Build history of the part. All positions in model axes, mm. A direction names the side the tool comes from. Round coordinates to 2 decimals unless told otherwise and drop trailing zeros. Loops run counter-clockwise (first coordinate to the right, second up) from the corner with the lowest first, then second, coordinate; pieces in that order, holes last.
from build123d import *

# Parameters (mm, degrees)
SKETCH1_W               = 150
SKETCH1_H               = 150
BOSS_EXTRUDE1_DEPTH     = 10
CUT_EXTRUDE1_DEPTH      = 3.1
CUT_EXTRUDE1_DEPTH_BACK = 3.1
CUT_EXTRUDE2_DEPTH      = 8.2
CUT_EXTRUDE2_DEPTH_BACK = 2
SKETCH4_W               = 24.2
SKETCH4_H               = 2


with BuildPart() as part:
    # Sketch1 → Boss-Extrude1 (new body)
    with BuildSketch(Plane(origin=(0, 0, 0), x_dir=(1, 0, 0), z_dir=(0, 1, 0))):
        Rectangle(SKETCH1_W, SKETCH1_H)
    extrude(amount=BOSS_EXTRUDE1_DEPTH)

    # Sketch3 → Cut-Extrude1 (cut, two sides: drawn at the far end of the back side and taken through both)
    with BuildSketch(Plane(origin=(0, 0, 0), x_dir=(0, -1, 0), z_dir=(0.7071067811865488, 0, 0.7071067811865464)).offset(-CUT_EXTRUDE1_DEPTH_BACK)):
        with BuildLine():
            Line((-4, -68.177876041), (-6, -68.177876041))
            ThreePointArc((-6, -68.177876041), (-6.294051831, -69.777876041), (-6, -71.377876041))
            Line((-6, -71.377876041), (-6, -75.277876041))
            Line((-6, -75.277876041), (-8, -75.277876041))
            Line((-8, -75.277876041), (-8, -65.077876041))
            Line((-8, -65.077876041), (-10, -65.077876041))
            Line((-10, -65.077876041), (-10, -89.277876041))
            Line((-10, -89.277876041), (-8, -89.277876041))
            Line((-8, -89.277876041), (-8, -83.277876041))
            Line((-8, -83.277876041), (-4, -83.277876041))
            Line((-4, -83.277876041), (-4, -71.377876041))
            ThreePointArc((-4, -71.377876041), (-3.705948169, -69.777876041), (-4, -68.177876041))
        make_face()
    extrude(amount=CUT_EXTRUDE1_DEPTH + CUT_EXTRUDE1_DEPTH_BACK, mode=Mode.SUBTRACT)

    # Sketch4 → Cut-Extrude2 (cut, two sides: drawn at the far end of the back side and taken through both)
    with BuildSketch(Plane(origin=(-2.192031022, 0, -2.192031022), x_dir=(0.7071067811865465, 0, -0.7071067811865487), z_dir=(0.7071067811865487, 0, 0.7071067811865465)).offset(-CUT_EXTRUDE2_DEPTH_BACK)):
        with Locations((-77.177876041, 9)):
            Rectangle(SKETCH4_W, SKETCH4_H)
    extrude(amount=CUT_EXTRUDE2_DEPTH + CUT_EXTRUDE2_DEPTH_BACK, mode=Mode.SUBTRACT)

    # Sketch5 → Revolve1 (revolve)
    with BuildSketch(Plane(origin=(0, 0, 0), x_dir=(0, -1, 0), z_dir=(0.7071067811865488, 0, 0.7071067811865464)), mode=Mode.PRIVATE) as revolve1_sk:
        with BuildLine():
            Line((-10, 46.066017178), (-35, 46.066017178))
            ThreePointArc((-35, 46.066017178), (-29.607626316, 53.030055538), (-21.31365255, 50.066017178))
            Line((-21.31365255, 50.066017178), (-10, 50.066017178))
            Line((-10, 50.066017178), (-10, 46.066017178))
        make_face()
    revolve(revolve1_sk.sketch.rotate(Axis((32.573593129, 36.96807126, -32.573593129), (0, -1, 0)), 135), axis=Axis((32.573593129, 36.96807126, -32.573593129), (0, -1, 0)))


solid = part.part
(1) Slice it at B-B on z = -6. List the corners of the cut face in (x, y), plus the area to 3 significant figures.
Responses:
outline: (-75, 0) - (75, 0) - (75, 10) - (-75, 10) - close
area: 1,500 mm2
(2) Pull direction X, two halves, no side cores. Call faces 4 (the face through (-75, 5, 1)), 5 (the face through (-49.355, 6.294, 49.294)), 6 (the face through (75, 5, 1)): +X half, -X half, draft (parallel to the pull), parting line (faces both ways), or undercut.
Responses:
face 4: -X half
face 5: undercut
face 6: +X half
(3) Slice it at C-C on y = 18. List the corners of the cut face in (x, z), plus the area to 3 significant figures.
Responses:
outline: circle Ø8 at (32.57, -32.57)
area: 50.3 mm2
(4) Slice it at A-A on x = 53. List the corners of the cut face in (y, z).
Responses:
outline: (0, -75) - (10, -75) - (10, 75) - (0, 75) - close
(5) Which spindle directions (+Z, -Z, +X, -X, +Y, -Y) get a long thin tool onto all of the face, cutting with end or side? Do faces 1 (the face through (-51.09, 9.01, 58.3)), 2 (the face through (-1, 0, -1)), 3 (the face through (28.608, 15.578, -33.094)). Say none if no direction does.
Responses:
face 1: +Y
face 2: +Z, -Z, +X, -X, -Y
face 3: none
(6) Pin check, flat tips, straight feed: P1, Ø8, axis at y = 17.5, z = -18.5, coming from the +X side; P2, Ø2, axis at x = -50.5, z = 51.5, coming from the -Y side; P3, Ø14, axis at x = -55, z = 55, coming from the +Y side; P4, Ø5, axis at x = 32.5, y = 27, coming from the -Z side. Stop position of each tip, or through.
Responses:
P1: passes through
P2: stops at y = 0
P3: stops at y = 10
P4: stops at z = -39.84
(7) Probe line 1 (Y direction, x = -45, z = -22); line 2 (X direction, y = 5, z = 60); line 3 (Y direction, x = -54, z = 58.5). List the from-to ranges inside material, lowest first.
Responses:
line 1: y = 0 to 10
line 2: x = -75 to -57.77, -55.62 to 75
line 3: y = 0 to 8
